Could you check a few things on this model? Use its own coordinates, in mm. A direction names the side the tool comes from. Coordinates: 2 decimals unless noted, no trailing zeros. Write each loop counter-clockwise with the first axis right and the second up, starting at its lowest first coordinate (ties: lowest second). Pieces come first, ordered by that corner, then holes. Notation, with made-up numbers: (53.5, -23) - (92.5, -23) arc R33 cw to (92.5, 8) - close; hole circle Ø5 at (-9, 19). An arc over 180 degrees is marked (long way). Answer as a JSON object with one key per item and string values. Group by question number.
1) If we section it at C-C (x = 0): Write out the boundary of the cut face in (y, z).
2) If we section it at A-A (z = 0): Write out the boundary of the cut face in (x, y).
3) If we section it at B-B (y = -7.5): Write out the boundary of the cut face in (x, z).
4) We'd pull the mould along X, two halves only. Please class faces 3 (the flat face through (6.801, -7.605, 23.521)), 4 (the cylindrical face through (30.5, -7.4, 20.5)), 5 (the cylindrical face through (-6.638, 2.535, 9.251)): released by +X, released by -X, zero draft, split by the parting line, or undercut.
5) Will these pins go through, and if not, where does the flat tip stop? pin 1 Ø7.5 at (y, z) = (-10, 8) entering from -X; pin 2 Ø4.5 at (x, z) = (8.49, -8.49) entering from -Y.
6) Please list where these lines run through material, in increasing order: line 1 along X through (y, z) = (3.85, 0); line 2 along Z through (x, y) = (26.5, -13.5); line 3 along Y through (x, z) = (30.15, -18).
7) On a 3-axis mill with a long thin cutter (end or side, diameter ignored), from which of +Z, -Z, +X, -X, +Y, -Y can I reach the whole of each face in a straight line? I mean faces 1 (the flat face through (28, -7, 0)), 2 (the flat face through (15, -3, 25)). Say none if no direction works.
8) If we section it at D-D (y = 2.5): Write out the boundary of the cut face in (x, z).
```python
from build123d import *

# Parameters (mm, degrees)
SKETCH1_W           = 30
SKETCH1_H           = 50
BOSS_EXTRUDE1_DEPTH = 5
SKETCH2_R           = 5
CUT_EXTRUDE1_DEPTH  = 5
SKETCH3_R           = 2
CUT_EXTRUDE2_DEPTH  = 10
SKETCH4_W           = 50
SKETCH4_H           = 5
BOSS_EXTRUDE2_DEPTH = 18
SKETCH5_W           = 50
SKETCH5_H           = 20
BOSS_EXTRUDE3_DEPTH = 5
SKETCH6_R           = 2.5
CUT_EXTRUDE3_DEPTH  = 5
BOSS_EXTRUDE4_DEPTH = 3


with BuildPart() as part:
    # Sketch1 → Boss-Extrude1 (new body)
    with BuildSketch(Plane(origin=(0, 0, 0), x_dir=(1, 0, 0), z_dir=(0, 1, 0))):
        Rectangle(SKETCH1_W, SKETCH1_H)
    extrude(amount=BOSS_EXTRUDE1_DEPTH)

    # Sketch2 → Cut-Extrude1 (cut)
    with BuildSketch(Plane(origin=(0, 5, 0), x_dir=(1, 0, 0), z_dir=(0, 1, 0))):
        Circle(SKETCH2_R)
    extrude(amount=-CUT_EXTRUDE1_DEPTH, mode=Mode.SUBTRACT)

    # Sketch3 → Cut-Extrude2 (cut)
    with BuildSketch(Plane(origin=(0, 5, 0), x_dir=(1, 0, 0), z_dir=(0, 1, 0))):
        with Locations((-8.485281374, 8.485281374)):
            Circle(SKETCH3_R)
        with Locations((8.485281374, 8.485281374)):
            Circle(SKETCH3_R)
        with Locations((-8.485281374, -8.485281374)):
            Circle(SKETCH3_R)
        with Locations((8.485281374, -8.485281374)):
            Circle(SKETCH3_R)
    extrude(amount=-CUT_EXTRUDE2_DEPTH, mode=Mode.SUBTRACT)

    # Sketch4 → Boss-Extrude2 (add)
    with BuildSketch(Plane(origin=(15, 0, 0), x_dir=(0, 0, -1), z_dir=(1, 0, 0))):
        with Locations((0, 2.5)):
            Rectangle(SKETCH4_W, SKETCH4_H)
    extrude(amount=BOSS_EXTRUDE2_DEPTH)

    # Sketch5 → Boss-Extrude3 (add)
    with BuildSketch(Plane(origin=(33, 0, 0), x_dir=(0, 0, -1), z_dir=(1, 0, 0))):
        with Locations((0, -5)):
            Rectangle(SKETCH5_W, SKETCH5_H)
    extrude(amount=-BOSS_EXTRUDE3_DEPTH)

    # Sketch6 → Cut-Extrude3 (cut)
    with BuildSketch(Plane(origin=(33, 0, 0), x_dir=(0, 0, -1), z_dir=(1, 0, 0))):
        with Locations((18, -7.5)):
            Circle(SKETCH6_R)
        with Locations((-18, -7.5)):
            Circle(SKETCH6_R)
    extrude(amount=-CUT_EXTRUDE3_DEPTH, mode=Mode.SUBTRACT)

    # Sketch7 → Boss-Extrude4 (add)
    with BuildSketch(Plane.XY.offset(25)):
        Polygon((28, -15), (-15, 0), (28, 0), align=None)
    boss_extrude4 = extrude(amount=-BOSS_EXTRUDE4_DEPTH)

    # Mirror1: Boss-Extrude4 across plane
    add(boss_extrude4.mirror(Plane.XY))


solid = part.part
```
Here are the results:
{
 "1": {"outline": "(-5.23, -25) - (5, -25) - (5, -5) - (0, -5) - (0, -22) - (-5.23, -22) - close; (-5.23, 22) - (0, 22) - (0, 5) - (5, 5) - (5, 25) - (-5.23, 25) - close"},
 "2": {"outline": "(-15, 0) - (-5, 0) - (-5, 5) - (-15, 5) - close; (5, 0) - (28, 0) - (28, -15) - (33, -15) - (33, 5) - (5, 5) - close"},
 "3": {"outline": "(6.5, -25) - (33, -25) - (33, -20.5) - (28, -20.5) - (28, -22) - (6.5, -22) - close; (6.5, 22) - (28, 22) - (28, 20.5) - (33, 20.5) - (33, 25) - (6.5, 25) - close; (28, -15.5) - (33, -15.5) - (33, 15.5) - (28, 15.5) - close"},
 "4": {"face 3": "released by -X", "face 4": "zero draft", "face 5": "undercut"},
 "5": {"pin 1": "stops at x = 28", "pin 2": "stops at y = 0"},
 "6": {"line 1": "x = -15 to -5, 5 to 33", "line 2": "z = -25 to -22, 22 to 25", "line 3": "y = -15 to -10, -5 to 5"},
 "7": {"face 1": "-X, -Y", "face 2": "+Z, +X, -X, +Y, -Y"},
 "8": {"outline": "(-15, -25) - (33, -25) - (33, 25) - (-15, 25) - close; hole circle Ø4 at (-8.49, -8.49); hole circle Ø4 at (-8.49, 8.49); hole circle Ø10 at (0, 0); hole circle Ø4 at (8.49, -8.49); hole circle Ø4 at (8.49, 8.49)"}
}
